Check sheet for the modelled part. Datum: model origin and axes. Units: mm. A direction names the side the tool comes from. Give positions to 0.01 mm unless a question says otherwise; leave off trailing zeros. Order: outer loops, then holes, each group sorted by start corner. A loop starts at its lowest first (then second) coordinate and runs counter-clockwise, first axis right, second up. Notation, with made-up numbers: M 87.25,21 L 100.25,21 A9 ccw 100.25,38 Z; hole C 61,20 d2. An arc over 180 degrees is marked long. Answer in a Markdown table with one row per item. Add a question column.
from build123d import *

# Parameters (mm, degrees)
FILLET1_R          = 2
CUT_EXTRUDE1_START = 37
CUT_EXTRUDE1_DEPTH = 10
CUT_EXTRUDE2_START = 22.5
CUT_EXTRUDE2_DEPTH = 10


with BuildPart() as part:
    # Sketch1 → Revolve1 (revolve)
    with BuildSketch(Plane(origin=(0, 0, 0), x_dir=(0, 0, -1), z_dir=(1, 0, 0))):
        Polygon((0, 0), (536, 0), (536, 32.5), (446, 32.5), (446, 35), (376, 35), (376, 37.5), (339, 37.5), (339, 42.5), (201.5, 42.5), (201.5, 45), (76.5, 45), (76.5, 55), (54, 55), (54, 42.5), (39, 42.5), (39, 37.5), (0, 37.5), align=None)
    revolve(axis=Axis((0, 0, 0), (0, 0, -1)))

    # Fillet1
    fillet1_edges = [part.edges().sort_by_distance(p)[0] for p in [
        (0, -37.5, 0),
        (0, -32.5, -536),
    ]]
    fillet(fillet1_edges, radius=FILLET1_R)

    # Sketch2 → Cut-Extrude1 (cut)
    with BuildSketch(Plane(origin=(0, 0, 0), x_dir=(1, 0, 0), z_dir=(0, 1, 0)).offset(CUT_EXTRUDE1_START)):
        with BuildLine():
            Line((9, 187.5), (9, 90.5))
            ThreePointArc((9, 90.5), (0, 81.5), (-9, 90.5))
            Line((-9, 90.5), (-9, 187.5))
            ThreePointArc((-9, 187.5), (0, 196.5), (9, 187.5))
        make_face()
    extrude(amount=CUT_EXTRUDE1_DEPTH, mode=Mode.SUBTRACT)

    # Sketch3 → Cut-Extrude2 (cut)
    with BuildSketch(Plane(origin=(0, 0, 0), x_dir=(1, 0, 0), z_dir=(0, 1, 0)).offset(CUT_EXTRUDE2_START)):
        with BuildLine():
            Line((10, 536), (10, 466))
            ThreePointArc((10, 466), (0, 456), (-10, 466))
            Line((-10, 466), (-10, 536))
            ThreePointArc((-10, 536), (0, 546), (10, 536))
        make_face()
    extrude(amount=CUT_EXTRUDE2_DEPTH, mode=Mode.SUBTRACT)


solid = part.part
Q1. Draft check along X on faces 1 (the cylindrical face through (0, 27, -456)), 2 (the cylindrical face through (-53.692, -11.923, -65.092)), 3 (the flat face through (-40, 21, -76.5)). Enter one of: pulls with the +X half, pulls with the -X half, needs draft (parallel to the pull), parting line crosses it, or undercut.
Q2. Cross-section at B-B (z = -101). Record the boundary of the cut face in (x, y), and give its area (3 significant figures).
Q3. Go/stop test with flat-tipped pins: pin 1 (10 mm diameter, centred on y = -32.5, z = -443, fed in from -X); pin 2 (10 mm diameter, centred on y = -18, z = -225.5, fed in from +X); pin 3 (6 mm diameter, centred on x = -27, z = -268, fed in from -Y). Record where each tip stops, or that it passes through.
Q4. Thickness scan on probe 1 along Z at (x, y) = (-48, 14); probe 2 along X at (y, z) = (-13, -406); probe 3 along Z at (x, y) = (-24.5, -28.5). Record the ranges inside material, lowest first.
Q5. Cross-section at A-A (z = -371.5). Record the boundary of the cut face in (x, y).
Q6. Tool access check on faces 4 (the flat face through (-23.2, -23.2, -446)), 5 (the cylindrical face through (-0.198, 40.944, -196.498)), 6 (the flat face through (-32.3, 28.3, -54)), 7 (the flat face through (0, 0, -536)). Record the directions out of +Z, -Z, +X, -X, +Y, -Y that give a thin tool (end or side, any length) a straight path to the whole face; none if there is none.
Values follow:
| question | item | result |
|---|---|---|
| 1 | face 1 | undercut |
| 1 | face 2 | parting line crosses it |
| 1 | face 3 | needs draft |
| 2 | outline | M -9,37 L -9,44.09 A45 ccw long 9,44.09 L 9,37 Z |
| 2 | area | 6,220 mm² |
| 3 | pin 1 | x = -21.65 |
| 3 | pin 2 | x = 40.46 |
| 3 | pin 3 | y = -35.07 |
| 4 | probe 1 | -76.5 to -54 |
| 4 | probe 2 | -32.5 to 32.5 |
| 4 | probe 3 | -339 to -39 |
| 5 | outline | C 0,0 d75 |
| 6 | face 4 | -Z |
| 6 | face 5 | +Y |
| 6 | face 6 | +Z |
| 6 | face 7 | -Z, +X, -X, +Y, -Y |
